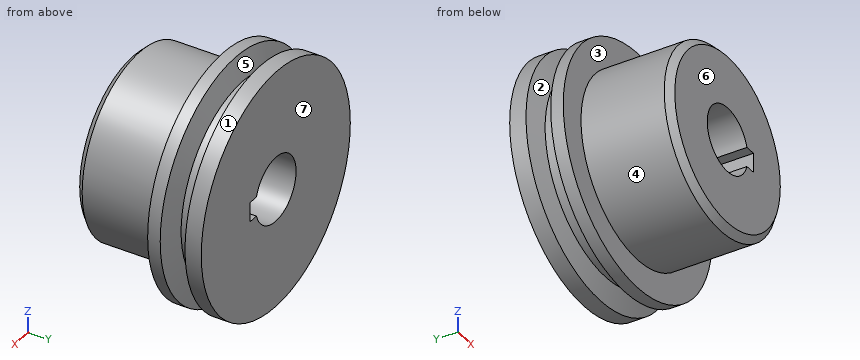
from build123d import *

# Parameters (mm, degrees)
SKETCH1_R           = 14
BOSS_EXTRUDE2_DEPTH = 22
CHAMFER1_SIZE       = 1


with BuildPart() as part:
    # Sketch1 → Boss-Extrude2 (new body)
    with BuildSketch(Plane(origin=(0, 0, 0), x_dir=(1, 0, 0), z_dir=(0, 1, 0))):
        Circle(SKETCH1_R)
        with BuildLine():
            Line((4.769696007, -1.5), (6.4, -1.5))
            Line((6.4, -1.5), (6.4, 1.5))
            Line((6.4, 1.5), (4.769696007, 1.5))
            ThreePointArc((4.769696007, 1.5), (-5, 0), (4.769696007, -1.5))
        make_face(mode=Mode.SUBTRACT)
    extrude(amount=BOSS_EXTRUDE2_DEPTH)

    # Chamfer1
    chamfer1_edges = [part.edges().sort_by_distance(p)[0] for p in [
        (-14, 0, 0),
    ]]
    chamfer(chamfer1_edges, length=CHAMFER1_SIZE)

    # Sketch2 → Revolve1 (revolve)
    with BuildSketch(Plane(origin=(0, 0, 0), x_dir=(0, 0, -1), z_dir=(1, 0, 0))):
        Polygon((14, 22), (18.362757193, 22), (18.362757193, 19.5), (15, 18.654420503), (15, 16.811960425), (18.362757193, 15.697914797), (18.362757193, 13.769758902), (14, 13.769758902), align=None)
    revolve(axis=Axis((0, 22, 0), (0, -1, 0)))


solid = part.part
Input: part model. Units: mm. Frame: model coordinates. Face numbers are marked on the shaded views. A direction names the side the tool comes from. Round coordinates to 2 decimals unless told otherwise and drop trailing zeros. Order: outer loops, then holes, each group sorted by start corner. A loop starts at its lowest first (then second) coordinate and runs counter-clockwise, first axis right, second up. Notation, with made-up numbers: (-34, 82.25) - (21, 82.25) arc R20 cw to (21, 105.25) - close; hole circle Ø8 at (0, 87). An arc over 180 degrees is marked (long way). Use a Markdown table: item, result.
1. Section A-A on x = 0. Return the cut outline in (y, z), then the cut area to 3 significant figures.
Evaluation:
| item | result |
|---|---|
| outline | (0, -13) - (1, -14) - (13.77, -14) - (13.77, -18.36) - (15.7, -18.36) - (16.81, -15) - (18.65, -15) - (19.5, -18.36) - (22, -18.36) - (22, -5) - (0, -5) - close; (0, 5) - (22, 5) - (22, 18.36) - (19.5, 18.36) - (18.65, 15) - (16.81, 15) - (15.7, 18.36) - (13.77, 18.36) - (13.77, 14) - (1, 14) - (0, 13) - close |
| area | 448 mm^2 |
2. Mould query, pull axis Y, two halves, no side actions, for the marked faces 4, 5, 6 and 7. Classes: +Y half, -Y half, draft (parallel to the pull), parting line (faces both ways), or undercut.
Evaluation:
| item | result |
|---|---|
| face 4 | draft |
| face 5 | undercut |
| face 6 | -Y half |
| face 7 | +Y half |
3. Material intervals for probe 1 along X at (y, z) = (15.5, 0); probe 2 along Z at (x, y) = (0, 12.5); probe 3 along X at (y, z) = (7, 0), sorted ascending.
Evaluation:
| item | result |
|---|---|
| probe 1 | -18.36 to -5, 6.4 to 18.36 |
| probe 2 | -14 to -5, 5 to 14 |
| probe 3 | -14 to -5, 6.4 to 14 |
4. Section B-B on z = 0. Return the cut outline in (x, y), then the cut area to 3 significant figures.
Evaluation:
| item | result |
|---|---|
| outline | (-18.36, 13.77) - (-14, 13.77) - (-14, 1) - (-13, 0) - (-5, 0) - (-5, 22) - (-18.36, 22) - (-18.36, 19.5) - (-15, 18.65) - (-15, 16.81) - (-18.36, 15.7) - close; (6.4, 0) - (13, 0) - (14, 1) - (14, 13.77) - (18.36, 13.77) - (18.36, 15.7) - (15, 16.81) - (15, 18.65) - (18.36, 19.5) - (18.36, 22) - (6.4, 22) - close |
| area | 417 mm^2 |
5. First-contact query: pin 1 (1.5 mm diameter, centred on x = 4, y = 9, fed in from +Z); pin 2 (3 mm diameter, centred on y = 14, z = -1.5, fed in from +X); pin 3 (0.5 mm diameter, centred on x = 5.5, y = 10.5, fed in from -Z); pin 4 (16 mm diameter, centred on x = 0, z = 0, fed in from -Y). Flat tips, straight axial feed; report the tip coordinate or a pass-through.
Evaluation:
| item | result |
|---|---|
| pin 1 | z = 13.62 |
| pin 2 | x = 18.36 |
| pin 3 | z = -12.98 |
| pin 4 | y = 0 |
6. Section C-C on y = 13.25. Return the cut outline in (x, z), then the cut area to 3 significant figures.
Evaluation:
| item | result |
|---|---|
| outline | circle Ø28 at (0, 0); hole (4.77, -1.5) - (6.4, -1.5) - (6.4, 1.5) - (4.77, 1.5) arc R5 ccw (long way) to start |
| area | 533 mm^2 |
7. Access query for the marked faces 1, 2 and 3. Directions: +Z, -Z, +X, -X, +Y, -Y. A direction counts if a zero-diameter tool reaches every point of the face in a straight line with its end or side. Return the directions, or none.
Evaluation:
| item | result |
|---|---|
| face 1 | +Y, -Y |
| face 2 | none |
| face 3 | -Y |
